Design review of the part built by this model. Coordinates are the model's own, in mm. Face numbers are marked on the shaded views. A direction names the side the tool comes from. Coordinates: 2 decimals unless noted, no trailing zeros. Loops run counter-clockwise (first coordinate to the right, second up) from the corner with the lowest first, then second, coordinate; pieces in that order, holes last. Notation, with made-up numbers: M 80,-7 L 93,-7 A16 ccw 93,22 Z; hole C 45,34 d4. An arc over 180 degrees is marked long. Answer as a JSON object with one key per item and string values. Group by question number.
1. Draft analysis for pull direction Z (two halves, no side actions). For the marked faces 3, 4 and 5, state which applies: +Z half, -Z half, draft (parallel to the pull), parting line (faces both ways), or undercut.
2. Consider section D-D (y = -4). State the section outline as (x, z) points, then the cut area to 3 significant figures.
3. Machinability: for the marked faces 1 and 2, which of the approach directions +Z, -Z, +X, -X, +Y, -Y give a long, thin tool a straight path to every point of the face, cutting with its end or side? Answer none if there is none.
4. Insertion check: pin 1 (4 mm diameter, centred on x = 3, z = -6, fed in from +Y); pin 2 (3 mm diameter, centred on x = 4, z = 0.5, fed in from +Y); pin 3 (1.5 mm diameter, centred on x = 1.5, y = -3, fed in from -Z). Each pin has a flat end and moves straight along its axis. Give the tip position at first contact, or say it passes through.
5. Consider section B-B (x = 9). State the section outline as (y, z) points.
6. To check wall thickness, follow probe 1 along X at (y, z) = (9.15, 0); probe 2 along X at (y, z) = (-11, 3.5); probe 3 along Y at (x, z) = (6.25, -1.75). State the ranges of each line that lie inside material, in increasing order.
7. Consider section C-C (z = 0). State the section outline as (x, y) points, then the cut area to 3 significant figures.
8. Consider section A-A (z = -4.5). State the section outline as (x, y) points.
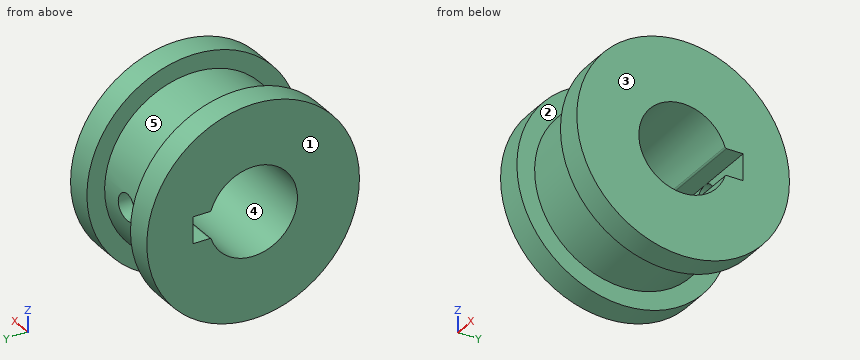
from build123d import *

# Parameters (mm, degrees)
SKETCH1_R               = 10
BOSS_EXTRUDE1_DEPTH     = 8
SKETCH3_R               = 12
BOSS_EXTRUDE2_DEPTH     = 3
SKETCH4_R               = 12
BOSS_EXTRUDE3_DEPTH     = 3
CUT_EXTRUDE2_DEPTH      = 3
CUT_EXTRUDE2_DEPTH_BACK = 11
SKETCH6_R               = 1.5
CUT_EXTRUDE3_DEPTH      = 5


with BuildPart() as part:
    # Sketch1 → Boss-Extrude1 (new body)
    with BuildSketch(Plane(origin=(0, 0, 0), x_dir=(0, 0, -1), z_dir=(1, 0, 0))):
        Circle(SKETCH1_R)
    extrude(amount=BOSS_EXTRUDE1_DEPTH)

    # Sketch3 → Boss-Extrude2 (add)
    with BuildSketch(Plane(origin=(8, 0, 0), x_dir=(0, 0, -1), z_dir=(1, 0, 0))):
        Circle(SKETCH3_R)
    extrude(amount=BOSS_EXTRUDE2_DEPTH)

    # Sketch4 → Boss-Extrude3 (add)
    with BuildSketch(Plane.ZY):
        Circle(SKETCH4_R)
    extrude(amount=BOSS_EXTRUDE3_DEPTH)

    # Sketch2 → Cut-Extrude2 (cut, two sides)
    with BuildSketch(Plane(origin=(8, 0, 0), x_dir=(0, 0, -1), z_dir=(1, 0, 0))) as cut_extrude2_sk:
        with BuildLine():
            Line((-1.5, 6.769696007), (1.5, 6.769696007))
            Line((1.5, 6.769696007), (1.5, 4.91426495))
            ThreePointArc((1.5, 4.91426495), (1.537093703, 4.79824108), (1.634615385, 4.72525476))
            ThreePointArc((1.634615385, 4.72525476), (0, -5), (-1.634615385, 4.72525476))
            ThreePointArc((-1.634615385, 4.72525476), (-1.537093703, 4.79824108), (-1.5, 4.91426495))
            Line((-1.5, 4.91426495), (-1.5, 6.769696007))
        make_face()
    extrude(amount=CUT_EXTRUDE2_DEPTH, mode=Mode.SUBTRACT)
    extrude(cut_extrude2_sk.sketch, amount=-CUT_EXTRUDE2_DEPTH_BACK, mode=Mode.SUBTRACT)

    # Sketch6 → Cut-Extrude3 (cut)
    with BuildSketch(Plane.XZ.offset(-6.769696007)):
        with Locations((4, 0)):
            Circle(SKETCH6_R)
    extrude(amount=-CUT_EXTRUDE3_DEPTH, mode=Mode.SUBTRACT)


solid = part.part
Findings below:
{
 "1": {"face 3": "draft", "face 4": "undercut", "face 5": "parting line"},
 "2": {"outline": "M -3,-11.31 L 0,-11.31 L 0,-9.17 L 8,-9.17 L 8,-11.31 L 11,-11.31 L 11,-3 L -3,-3 Z; M -3,3 L 11,3 L 11,11.31 L 8,11.31 L 8,9.17 L 0,9.17 L 0,11.31 L -3,11.31 Z", "area": "198 mm^2"},
 "3": {"face 1": "+Z, -Z, -X, +Y, -Y", "face 2": "none"},
 "4": {"pin 1": "stops at y = 9.17", "pin 2": "stops at y = 10", "pin 3": "stops at z = -9.74"},
 "5": {"outline": "C 0,0 d24; hole M 4.73,-1.63 A0.2 cw 4.91,-1.5 L 6.77,-1.5 L 6.77,1.5 L 4.91,1.5 A0.2 cw 4.73,1.63 A5 ccw long Z"},
 "6": {"probe 1": "x = -3 to 2.5, 5.5 to 11", "probe 2": "x = -3 to 0, 8 to 11", "probe 3": "y = -9.85 to -4.68, 4.68 to 9.85"},
 "7": {"outline": "M -3,-12 L 0,-12 L 0,-10 L 8,-10 L 8,-12 L 11,-12 L 11,-5 L -3,-5 Z; M -3,6.77 L 2.5,6.77 L 2.5,10 L 0,10 L 0,12 L -3,12 Z; M 5.5,6.77 L 11,6.77 L 11,12 L 8,12 L 8,10 L 5.5,10 Z", "area": "130 mm^2"},
 "8": {"outline": "M -3,-11.12 L 0,-11.12 L 0,-8.93 L 8,-8.93 L 8,-11.12 L 11,-11.12 L 11,-2.18 L -3,-2.18 Z; M -3,2.18 L 11,2.18 L 11,11.12 L 8,11.12 L 8,8.93 L 0,8.93 L 0,11.12 L -3,11.12 Z"}
}
